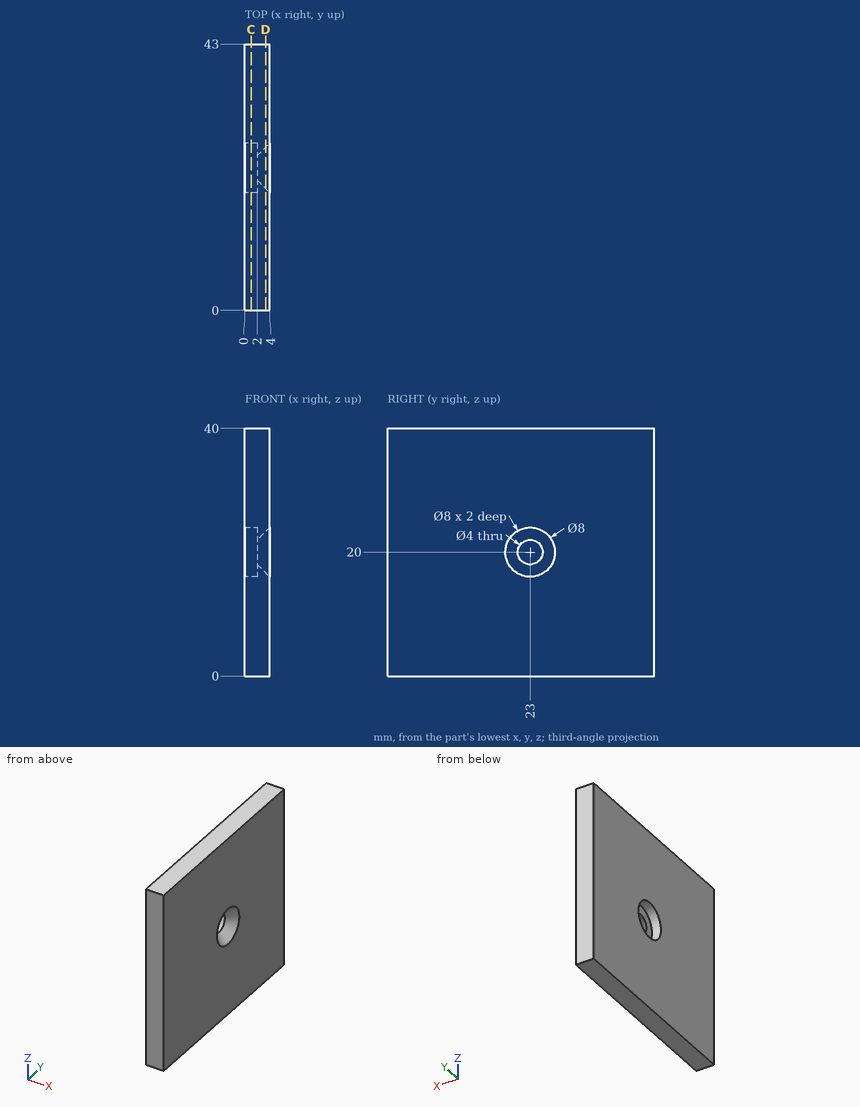
The drawing under review shows one solid part. Ordinate dimensions are in mm from its lowest x, y, z. Round coordinates to 2 decimals unless told otherwise and drop trailing zeros. Write each loop counter-clockwise with the first axis right and the second up, starting at its lowest first coordinate (ties: lowest second). Pieces come first, ordered by that corner, then holes.
(1) We need section D-D on x = 3.35. Give the boundary of the cut face in (y, z).
(2) Wall thickness on L1, parallel to Y at x = 0.9, z = 20; L2, parallel to Y at x = 2.05, z = 20; L3, parallel to Z at x = 0.3, y = 20 (1 decimal): over which ranges is each line inside the solid? List them lowest first.
(3) Insertion check: pin 1 (2.5 mm diameter, centred on y = 22, z = 20, fed in from -X); pin 2 (7 mm diameter, centred on y = 23, z = 20, fed in from +X). Each pin has a flat end and moves straight along its axis. Give the tip position at first contact, or say it passes through.
(4) We need section C-C on x = 1. Give the boundary of the cut face in (y, z).
Findings below:
1. outline: (0, 0) - (43, 0) - (43, 40) - (0, 40) - close; hole circle Ø6.7 at (23, 20)
2. L1: y = 0 to 19, 27 to 43
2. L2: y = 0 to 20.95, 25.05 to 43
2. L3: z = 0 to 17.4, 22.6 to 40
3. pin 1: stops at x = 2
3. pin 2: stops at x = 3.5
4. outline: (0, 0) - (43, 0) - (43, 40) - (0, 40) - close; hole circle Ø8 at (23, 20)
